Can you work these out from the model? Positions are in its coordinate system, mm. A direction names the side the tool comes from. Round coordinates to 2 decimals unless told otherwise and drop trailing zeros. Order: outer loops, then holes, each group sorted by start corner. A loop starts at its lowest first (then second) coordinate and runs counter-clockwise, first axis right, second up.
Q1. For faces 5 (the face through (4, 3, -59)), 6 (the face through (99, 4, 0)), 7 (the face through (198, 5.35, -60)), which set-ups out of +Z, -Z, +X, -X, +Y, -Y let a thin tool reach every point of the face, with its end or its side?
Q2. If we section it at C-C (z = -18.5): Please give me the cut outline in (x, y), plus the area to 3 significant figures.
Q3. If we section it at A-A (z = -74): Please give me the cut outline in (x, y), plus the area to 3 significant figures.
Q4. We'd pull the mould along X, two halves only. Please class faces 1 (the face through (0, 3, -59)), 2 (the face through (198, 3.35, -60)), 3 (the face through (200, 3, -59)), 4 (the face through (191, 4, -98.5)): pulls with the +X half, pulls with the -X half, needs draft (parallel to the pull), parting line crosses it, or undercut.
Q5. If we section it at B-B (x = 102.5): Please give me the cut outline in (y, z), plus the area to 3 significant figures.
Q6. Will these pins go through, and if not, where does the flat tip stop? P1, Ø4, axis at x = 113.5, y = 4, coming from the +Z side; P2, Ø1.2, axis at y = 8, z = -111, coming from the +X side.
Q7. If I drill on line 1 (Z direction, x = 126, y = 2); line 2 (X direction, y = 3.25, z = -16); line 3 (X direction, y = 2.5, z = -51), over which ranges is the centre line in solid material (lowest first)?
from build123d import *

# Parameters (mm, degrees)
SKETCH8_W           = 200
SKETCH8_H           = 120
SKETCH8_R           = 2.35
BOSS_EXTRUDE4_DEPTH = 1.35
SKETCH9_W           = 200
SKETCH9_H           = 120
SKETCH9_R           = 2.35
BOSS_EXTRUDE5_DEPTH = 6
SKETCH10_W          = 0.8
SKETCH10_H          = 8.103385626
SKETCH10_W_2        = 166.613370644
SKETCH10_H_2        = 0.8
SKETCH10_H_3        = 70.515232796
BOSS_EXTRUDE6_DEPTH = 1.05
CUT_EXTRUDE1_REACH  = 235.389
CUT_EXTRUDE2_REACH  = 235.389


with BuildPart() as part:
    # Sketch8 → Boss-Extrude4 (new body)
    with BuildSketch(Plane(origin=(0, 0, 0), x_dir=(1, 0, 0), z_dir=(0, 1, 0))):
        with Locations((100, 60)):
            Rectangle(SKETCH8_W, SKETCH8_H)
        with Locations(Location((5.806188151, 6.51599975, 0), (0, 0, 90))):
            Circle(SKETCH8_R, mode=Mode.SUBTRACT)
        with Locations(Location((194.233048897, 6.51599975, 0), (0, 0, 90))):
            Circle(SKETCH8_R, mode=Mode.SUBTRACT)
        with Locations(Location((194.233048897, 114.215856496, 0), (0, 0, 90))):
            Circle(SKETCH8_R, mode=Mode.SUBTRACT)
        with Locations(Location((5.806188151, 114.215856496, 0), (0, 0, 90))):
            Circle(SKETCH8_R, mode=Mode.SUBTRACT)
        Polygon((2.75, 95.557616398), (2.75, 24.442383602), (3.85, 24.442383602), (3.85, 21.35), (13.85, 21.35), (13.85, 14.747824367), (12.75, 14.747824367), (12.75, 6.044438741), (13.85, 6.044438741), (13.85, 3.35), (16.393314678, 3.35), (16.393314678, 2.25), (183.606685322, 2.25), (183.606685322, 3.35), (186.15, 3.35), (186.15, 6.044438741), (187.25, 6.044438741), (187.25, 14.747824367), (186.15, 14.747824367), (186.15, 21.35), (196.15, 21.35), (196.15, 24.442383602), (197.25, 24.442383602), (197.25, 95.557616398), (196.15, 95.557616398), (196.15, 98.65), (186.15, 98.65), (186.15, 105.252175633), (187.25, 105.252175633), (187.25, 113.955561259), (186.15, 113.955561259), (186.15, 116.65), (183.606685322, 116.65), (183.606685322, 117.75), (16.393314678, 117.75), (16.393314678, 116.65), (13.85, 116.65), (13.85, 113.955561259), (12.75, 113.955561259), (12.75, 105.252175633), (13.85, 105.252175633), (13.85, 98.65), (3.85, 98.65), (3.85, 95.557616398), align=None, mode=Mode.SUBTRACT)
    extrude(amount=BOSS_EXTRUDE4_DEPTH)

    # Sketch9 → Boss-Extrude5 (add)
    with BuildSketch(Plane(origin=(0, 1.35, 0), x_dir=(1, 0, 0), z_dir=(0, 1, 0))):
        with Locations((100, 60)):
            Rectangle(SKETCH9_W, SKETCH9_H)
        with Locations(Location((194.233048897, 114.215856496, 0), (0, 0, 90))):
            Circle(SKETCH9_R, mode=Mode.SUBTRACT)
        with Locations(Location((194.233048897, 6.51599975, 0), (0, 0, 90))):
            Circle(SKETCH9_R, mode=Mode.SUBTRACT)
        with Locations(Location((5.806188151, 6.51599975, 0), (0, 0, 90))):
            Circle(SKETCH9_R, mode=Mode.SUBTRACT)
        with Locations(Location((5.806188151, 114.215856496, 0), (0, 0, 90))):
            Circle(SKETCH9_R, mode=Mode.SUBTRACT)
        Polygon((183.456685322, 116.5), (186, 116.5), (186, 113.805561259), (186, 105.402175633), (186, 98.5), (196, 98.5), (196, 95.407616398), (196, 24.592383602), (196, 21.5), (186, 21.5), (186, 14.597824367), (186, 6.194438741), (186, 3.5), (183.456685322, 3.5), (16.543314678, 3.5), (14, 3.5), (14, 6.194438741), (14, 14.597824367), (14, 21.5), (4, 21.5), (4, 24.592383602), (4, 95.407616398), (4, 98.5), (14, 98.5), (14, 105.402175633), (14, 113.805561259), (14, 116.5), (16.543314678, 116.5), align=None, mode=Mode.SUBTRACT)
    extrude(amount=BOSS_EXTRUDE5_DEPTH)

    # Sketch10 → Boss-Extrude6 (add)
    with BuildSketch(Plane(origin=(0, 7.35, 0), x_dir=(1, 0, 0), z_dir=(0, 1, 0))):
        with Locations((13.45, 109.603868446)):
            Rectangle(SKETCH10_W, SKETCH10_H)
        with Locations((186.55, 109.603868446)):
            Rectangle(SKETCH10_W, SKETCH10_H)
        with Locations((100, 117.05)):
            Rectangle(SKETCH10_W_2, SKETCH10_H_2)
        with Locations((196.55, 60)):
            Rectangle(SKETCH10_W, SKETCH10_H_3)
        with Locations((186.55, 10.396131554)):
            Rectangle(SKETCH10_W, SKETCH10_H)
        with Locations((100, 2.95)):
            Rectangle(SKETCH10_W_2, SKETCH10_H_2)
        with Locations((13.45, 10.396131554)):
            Rectangle(SKETCH10_W, SKETCH10_H)
        with Locations((3.45, 60)):
            Rectangle(SKETCH10_W, SKETCH10_H_3)
    extrude(amount=BOSS_EXTRUDE6_DEPTH)

    # Sketch11 → Cut-Extrude1 (cut, up to next)
    with BuildSketch(Plane.ZY, mode=Mode.PRIVATE) as cut_extrude1_sk1:
        with BuildLine():
            Line((-60.5, 3.35), (-59.5, 3.35))
            ThreePointArc((-59.5, 3.35), (-58.5, 4.35), (-59.5, 5.35))
            Line((-59.5, 5.35), (-60.5, 5.35))
            ThreePointArc((-60.5, 5.35), (-61.5, 4.35), (-60.5, 3.35))
        make_face()
    cut_extrude1_tool1 = extrude(cut_extrude1_sk1.sketch, amount=-CUT_EXTRUDE1_REACH, mode=Mode.PRIVATE) & part.part
    add(cut_extrude1_tool1.solids().sort_by_distance((0, 4.35, -60))[0], mode=Mode.SUBTRACT)

    # Sketch12 → Cut-Extrude2 (cut, up to next)
    with BuildSketch(Plane(origin=(200, 0, 0), x_dir=(0, 0, -1), z_dir=(1, 0, 0)), mode=Mode.PRIVATE) as cut_extrude2_sk1:
        with BuildLine():
            Line((58, 5.35), (62, 5.35))
            ThreePointArc((62, 5.35), (63, 4.35), (62, 3.35))
            Line((62, 3.35), (58, 3.35))
            ThreePointArc((58, 3.35), (57, 4.35), (58, 5.35))
        make_face()
    cut_extrude2_tool1 = extrude(cut_extrude2_sk1.sketch, amount=-CUT_EXTRUDE2_REACH, mode=Mode.PRIVATE) & part.part
    add(cut_extrude2_tool1.solids().sort_by_distance((200, 4.35, -60))[0], mode=Mode.SUBTRACT)


solid = part.part
Solution:
1. face 5: +Y, -Y
1. face 6: +Z, +X, -X, +Y, -Y
1. face 7: +X
2. outline: (0, 0) - (13.85, 0) - (13.85, 1.35) - (14, 1.35) - (14, 7.35) - (0, 7.35) - close; (186, 1.35) - (186.15, 1.35) - (186.15, 0) - (200, 0) - (200, 7.35) - (186, 7.35) - close
2. area: 205 mm2
3. outline: (0, 0) - (2.75, 0) - (2.75, 1.35) - (4, 1.35) - (4, 7.35) - (3.85, 7.35) - (3.85, 8.4) - (3.05, 8.4) - (3.05, 7.35) - (0, 7.35) - close; (196, 1.35) - (197.25, 1.35) - (197.25, 0) - (200, 0) - (200, 7.35) - (196.95, 7.35) - (196.95, 8.4) - (196.15, 8.4) - (196.15, 7.35) - (196, 7.35) - close
3. area: 57.1 mm2
4. face 1: pulls with the -X half
4. face 2: needs draft
4. face 3: pulls with the +X half
4. face 4: undercut
5. outline: (0, -120) - (7.35, -120) - (7.35, -117.45) - (8.4, -117.45) - (8.4, -116.65) - (7.35, -116.65) - (7.35, -116.5) - (1.35, -116.5) - (1.35, -117.75) - (0, -117.75) - close; (0, -2.25) - (1.35, -2.25) - (1.35, -3.5) - (7.35, -3.5) - (7.35, -3.35) - (8.4, -3.35) - (8.4, -2.55) - (7.35, -2.55) - (7.35, 0) - (0, 0) - close
5. area: 49.8 mm2
6. P1: stops at z = 0
6. P2: stops at x = 186.95
7. line 1: z = -120 to -116.5, -3.5 to 0
7. line 2: x = 0 to 14, 186 to 200
7. line 3: x = 0 to 4, 196 to 200
